Work out the finished part from the listing and answer in its coordinate system (mm). A direction names the side the tool comes from. Coordinates: 2 decimals unless noted, no trailing zeros. Order: outer loops, then holes, each group sorted by start corner. A loop starts at its lowest first (then second) coordinate and runs counter-clockwise, first axis right, second up. Notation, with made-up numbers: (-20, 6.25) - (31, 6.25) arc R32 cw to (31, 40.25) - close; hole circle Ø2 at (88.25, 24). An arc over 180 degrees is marked (long way). Answer as a JSON object with one key per item and string values. Group by question number.
1) Section C-C (z = 26.5) is taken. Count the separate pieces of the cut face and the enclosed holes in it, plus the area to 3 significant figures.
2) The mould has two halves that part along Z. Classify faces 6 (the face through (67.914, -29, 34)), 7 (the face through (-4, 9.7, 79.7)), 8 (the face through (16, 46, 9.181)): released by +Z, released by -Z, zero draft, split by the parting line, or undercut.
3) A tool of negligible diameter and unlimited length cuts with its end or side. For faces 1 (the face through (39, 31.242, 24)), 2 (the face through (35.269, 36, 22)), 3 (the face through (0, 1, 74)), 4 (the face through (64, -34, 68.834)), 5 (the face through (-1, -1, -20.549)), from which of +Z, -Z, +X, -X, +Y, -Y can it reach the whole face along a straight path? Write none if from no direction.
4) Each of these flat-tipped pins is pushed along its axis until it touches: P1, Ø12, axis at y = 3, z = 76.5, coming from the -X side; P2, Ø10, axis at x = -2, y = -61, coming from the +Z side; P3, Ø5.5, axis at x = 11.08, z = 51.15, coming from the -Y side. Where does it stop, or does it pass through?
5) Section A-A (x = -14.5) is taken. Give the vertices of the cut face in (y, z).
6) Find the intervals of material crossed by line 1 along X through (y, z) = (-23, 34); line 2 along Y through (x, z) = (-3, 33); line 3 along X through (y, z) = (-35.5, 52.5), in increasing order.
7) Section B-B (y = -5.5) is taken. Give the vertices of the cut face in (x, z).
from build123d import *

# Parameters (mm, degrees)
F0_W          = 153.0245915055
F0_H          = 20.5490160733
F1_DEPTH      = 75.946
F1_DEPTH_BACK = 75.946
F3_DEPTH      = 68.834
F5_START      = -31.242
F4_W          = 31.1878696084
F4_H          = 3.7891790271
F4_W_2        = 30.604918953
F4_H_2        = 9.1814752668
F5_DEPTH      = 38.862
F7_START      = -39.37
F6_R          = 4.5342929644
F6_R_2        = 4.5529905845
F7_DEPTH      = 30.734
F8_W          = 7.8698322177
F8_H          = 124.7514784336
F9_DEPTH      = 69.088
F10_W         = 3.4977030009
F10_H         = 13.4078674018
F11_DEPTH     = 68.834
F12_W         = 4.9550831318
F12_H         = 39.0577064827
F12_W_2       = 39.0577036887
F12_H_2       = 7.869835943
F13_DEPTH     = 68.834
F15_START     = 38.608
F15_DEPTH     = 30.988
F16_W         = 9.7991945222
F16_H         = 10.9250182286
F16_W_2       = 12.1427290142
F16_H_2       = 10.8340159059
F16_W_3       = 14.9299055338
F16_H_3       = 13.1014734507
F16_W_4       = 13.116395101
F16_H_4       = 12.3132541776
F17_DEPTH     = 78.74
F19_DEPTH     = 8.128
F20_R         = 10.030835309
F20_R_2       = 7.2175731122
F21_DEPTH     = 133.096
F22_W         = 29.4703273103
F22_H         = 0.956825912
F23_DEPTH     = 0.254


with BuildPart() as f1:
    # F0 (on Front) → F1 (new body, two sides)
    with BuildSketch(Plane.XZ) as f1_sk:
        with Locations((-0.1457370818, -10.2745080367)):
            Rectangle(F0_W, F0_H)
    extrude(amount=F1_DEPTH)
    extrude(f1_sk.sketch, amount=-F1_DEPTH_BACK)

    # F2 (on face) → F3 (join)
    with BuildSketch(Plane.XY):
        Polygon((69.0796747804, 69.8083639145), (4.0806569159, 69.8083639145), (69.0796747804, 10.9303286299), align=None)
    extrude(amount=F3_DEPTH)

    # F4 (on Front) → F5 (join)
    with BuildSketch(Plane.XZ.offset(F5_START)):
        with Locations((19.6745917201, 36.4344269037)):
            Rectangle(F4_W, F4_H)
        Polygon((35.2685265243, 61.0640980303), (35.2685265243, 38.3290164173), (35.2685265243, 34.5398373902), (35.2685265243, 9.1814752668), (35.2685265243, 0), (68.7882006168, 0), (68.7882006168, 61.0640980303), align=None)
        with Locations((19.9660670478, 4.5907376334)):
            Rectangle(F4_W_2, F4_H_2)
    extrude(amount=-F5_DEPTH)

    # F6 (on Front) → F7 (join)
    with BuildSketch(Plane.XZ.offset(F7_START)):
        with BuildLine():
            ThreePointArc((13.2766587373, 44.7414778173), (16.5933676498, 47.2141890003), (17.8556101724, 51.153935492))
            ThreePointArc((17.8556101724, 51.153935492), (7.13631922, 56.6712374301), (8.875472686, 44.7414778173))
            Line((8.875472686, 44.7414778173), (13.2766587373, 44.7414778173))
        make_face()
        with Locations((11.0760657117, 51.153935492)):
            Circle(F6_R, mode=Mode.SUBTRACT)
        with BuildLine():
            Line((13.2766587373, 44.7414778173), (8.875472686, 44.7414778173))
            ThreePointArc((8.875472686, 44.7414778173), (11.0760657117, 44.3743910313), (13.2766587373, 44.7414778173))
        make_face()
        with BuildLine():
            ThreePointArc((13.2766587373, 44.7414778173), (11.0760657117, 44.3743910313), (8.875472686, 44.7414778173))
            Line((8.875472686, 44.7414778173), (3.7891815882, 44.7414778173))
            Line((3.7891815882, 44.7414778173), (3.7891815882, 38.9119684696))
            Line((3.7891815882, 38.9119684696), (17.7800003439, 38.9119684696))
            Line((17.7800003439, 38.9119684696), (17.7800003439, 44.7414778173))
            Line((17.7800003439, 44.7414778173), (13.2766587373, 44.7414778173))
        make_face()
        with BuildLine():
            Line((24.4199383292, 44.7414778173), (17.7800003439, 44.7414778173))
            Line((17.7800003439, 44.7414778173), (17.7800003439, 38.9119684696))
            Line((17.7800003439, 38.9119684696), (35.2685265243, 38.9119684696))
            Line((35.2685265243, 38.9119684696), (35.2685265243, 44.7414778173))
            Line((35.2685265243, 44.7414778173), (29.7944870558, 44.7414778173))
            ThreePointArc((29.7944870558, 44.7414778173), (27.1072126925, 44.2011621652), (24.4199383292, 44.7414778173))
        make_face()
        with BuildLine():
            Line((29.7944870558, 44.7414778173), (24.4199383292, 44.7414778173))
            ThreePointArc((24.4199383292, 44.7414778173), (27.1072126925, 44.2011621652), (29.7944870558, 44.7414778173))
        make_face()
        with BuildLine():
            ThreePointArc((34.0599860193, 51.153935492), (23.256430472, 56.9429365479), (24.4199383292, 44.7414778173))
            Line((24.4199383292, 44.7414778173), (29.7944870558, 44.7414778173))
            ThreePointArc((29.7944870558, 44.7414778173), (32.8962137483, 47.3031532716), (34.0599860193, 51.153935492))
        make_face()
        with Locations((27.1072126925, 51.153935492)):
            Circle(F6_R_2, mode=Mode.SUBTRACT)
    extrude(amount=-F7_DEPTH)

    # F8 (on Top) → F9 (join)
    with BuildSketch(Plane.XY):
        Polygon((-55.0888516009, 69.8083639145), (68.7882006168, 69.8083639145), (76.6580328345, 69.8083639145), (76.6580328345, 76.2208253145), (-55.0888516009, 76.2208253145), align=None)
        with Locations((72.7231167257, 7.4326246977)):
            Rectangle(F8_W, F8_H)
    extrude(amount=F9_DEPTH)

    # F10 (on Top) → F11 (join)
    with BuildSketch(Plane.XY):
        Polygon((67.9137706757, -19.9660658836), (67.9137706757, -2.7690164279), (60.9183646739, -2.7690164279), (60.9183646739, -19.9660658836), (64.4160676748, -19.9660658836), align=None)
        with Locations((66.1649191752, -26.6699995846)):
            Rectangle(F10_W, F10_H)
        Polygon((67.9137706757, -54.0686920285), (67.9137706757, -33.3739332855), (64.4160676748, -33.3739332855), (57.1291781962, -33.3739332855), (57.1291781962, -54.0686920285), align=None)
    extrude(amount=F11_DEPTH)

    # F12 (on Top) → F13 (join)
    with BuildSketch(Plane.XY):
        Polygon((76.366558671, -60.4811497033), (76.366558671, -54.3601661921), (4.9550831318, -54.3601661921), (0, -54.3601661921), (0, -60.4811497033), align=None)
        with Locations((2.4775415659, -34.8313129507)):
            Rectangle(F12_W, F12_H)
        Polygon((-47.2190156579, 75.9293437004), (-55.0888516009, 75.9293437004), (-55.0888516009, 21.4234422892), (-47.2190156579, 21.4234422892), (-47.2190156579, 29.2932782322), align=None)
        with Locations((-27.6901638135, 25.3583602607)):
            Rectangle(F12_W_2, F12_H_2)
    extrude(amount=F13_DEPTH)

    # F14 (on face) → F15 (join)
    with BuildSketch(Plane.XY.offset(F15_START)):
        Polygon((4.9550831318, -15.3024597093), (-8.1613119692, 29.2932782322), (-8.1613119692, 21.4234422892), (0, -15.3024597093), align=None)
    extrude(amount=F15_DEPTH)

    # F16 (on face) → F17 (join)
    with BuildSketch(Plane.XY):
        with Locations((0.0554858707, -18.9537699334)):
            Rectangle(F16_W, F16_H)
        with Locations((-14.2326764762, 23.8762702793)):
            Rectangle(F16_W_2, F16_H_2)
        with Locations((-54.6839684248, 22.7425415069)):
            Rectangle(F16_W_3, F16_H_3)
        with Locations((-1.6031144187, -60.5167932808)):
            Rectangle(F16_W_4, F16_H_4)
    extrude(amount=F17_DEPTH)

    # F18 (on Right) → F19 (join)
    with BuildSketch(Plane.YZ):
        Polygon((15.8831458539, 70.4239010811), (16.1645952612, 76.8972411752), (11.3799506798, 76.8972411752), (8.0025549978, 82.5262367725), (4.6251597814, 85.3407308459), (2.2797496705, 82.5262367725), (-2.4110814556, 76.8972411752), (-14.2319686711, 76.8972411752), (-14.2319686711, 70.4239010811), align=None)
    extrude(amount=-F19_DEPTH)

    # F20 (on Top) → F21 (join)
    with BuildSketch(Plane.XY):
        with Locations((-64.4248649478, -47.9438453913)):
            Circle(F20_R)
        with Locations((-64.4248649478, -47.9438453913)):
            Circle(F20_R_2, mode=Mode.SUBTRACT)
    extrude(amount=F21_DEPTH)

    # F22 (on Right) → F23 (join)
    with BuildSketch(Plane.YZ):
        Polygon((16.2943303585, 69.6600824594), (16.2943303585, 76.9319757819), (15.2609543875, 76.9319757819), (15.2609543875, 70.6169083714), (15.2609543875, 69.6600824594), align=None)
        with Locations((0.5257907324, 70.1384954154)):
            Rectangle(F22_W, F22_H)
    extrude(amount=-F23_DEPTH)


solid = f1.part
Report:
{
 "1": {"separate pieces": "3", "enclosed holes": "1", "area": "6,030 mm²"},
 "2": {"face 6": "zero draft", "face 7": "released by +Z", "face 8": "undercut"},
 "3": {"face 1": "+Z", "face 2": "none", "face 3": "+Z, +X, +Y", "face 4": "+Z, -Y", "face 5": "-Z, +X, -X, +Y, -Y"},
 "4": {"P1": "stops at x = -8.13", "P2": "stops at z = 78.74", "P3": "stops at y = -60.48"},
 "5": {"outline": "(-75.95, -20.55) - (75.95, -20.55) - (75.95, 0) - (76.22, 0) - (76.22, 69.09) - (69.81, 69.09) - (69.81, 0) - (29.29, 0) - (29.29, 78.74) - (18.46, 78.74) - (18.46, 0) - (-75.95, 0) - close"},
 "6": {"line 1": "x = -4.84 to 4.96, 64.42 to 67.91, 68.79 to 76.66", "line 2": "y = -66.67 to -54.36, -24.42 to -13.49, 69.81 to 76.22", "line 3": "x = 0 to 4.96, 57.13 to 67.91, 68.79 to 76.66"},
 "7": {"outline": "(-76.66, -20.55) - (76.37, -20.55) - (76.37, 0) - (76.66, 0) - (76.66, 69.09) - (68.79, 69.09) - (68.79, 0) - (67.91, 0) - (67.91, 68.83) - (60.92, 68.83) - (60.92, 0) - (-76.66, 0) - close; (-8.13, 70.42) - (-0.25, 70.42) - (-0.25, 69.66) - (0, 69.66) - (0, 76.9) - (-8.13, 76.9) - close; (-2.18, 38.61) - (2.07, 38.61) - (2.07, 69.6) - (-2.18, 69.6) - close"}
}
